```python
from build123d import *

# Parameters (mm, degrees)
CROQUIS3_R              = 6.25
CROQUIS3_R_2            = 4.25
SALIENTE_EXTRUIR1_DEPTH = 12
CORTAR_EXTRUIR1_DEPTH   = 10


with BuildPart() as part:
    # Croquis2 → Revolución1 (revolve)
    with BuildSketch(Plane.XY):
        Polygon((-4.25, 0), (-8, 7.5), (-10, 7.5), (-6.25, 0), align=None)
    revolve(axis=Axis((0, 7.5, 0), (0, -1, 0)))

    # Croquis3 → Saliente-Extruir1 (add)
    with BuildSketch(Plane.XZ):
        Circle(CROQUIS3_R)
        Circle(CROQUIS3_R_2, mode=Mode.SUBTRACT)
    extrude(amount=SALIENTE_EXTRUIR1_DEPTH)

    # Croquis4 → Cortar-Extruir1 (cut)
    with BuildSketch(Plane(origin=(0, 7.5, 0), x_dir=(1, 0, 0), z_dir=(0, 1, 0))):
        Polygon((-10.977061444, 8), (10.977061444, 8), (0, 12.60914387), align=None)
    extrude(amount=-CORTAR_EXTRUIR1_DEPTH, mode=Mode.SUBTRACT)


solid = part.part
```
The model under review builds one solid part; all positions refer to its coordinate system, in mm. A direction names the side the tool comes from. Give positions to 0.01 mm unless a question says otherwise; leave off trailing zeros. Write each loop counter-clockwise with the first axis right and the second up, starting at its lowest first coordinate (ties: lowest second). Pieces come first, ordered by that corner, then holes. Notation, with made-up numbers: M -23.5,-25.75 L 19.5,-25.75 A20 cw 19.5,-20.75 Z; hole C -24,40 d7. An arc over 180 degrees is marked long. Write each question's results on one line, items separated by ' | '. Start each with the question number.
1. For probe 1 along X at (y, z) = (-9.25, 0); probe 2 along X at (y, z) = (6.25, -1.25), list the stretches that pass through material, from the lowest coordinate up. Write a range as [from, to].
2. We need section A-A (z = 0). Write out the cut boundary in (x, y).
3. We need section B-B (y = -10.25). Write out the cut boundary in (x, z).
4. For faces 4 (the cylindrical face through (2.285, -5.916, 3.584)), 5 (the cylindrical face through (5.96, -5.92, 1.88)), list the 3-axis set-ups (+Z, -Z, +X, -X, +Y, -Y) from which the entire face can be reached by the end or side of a thin tool; tool diameter is ignored.
5. We need section C-C (y = 2.75). Write out the cut boundary in (x, z) (3 decimals), and give its area (3 significant figures).
6. Mouldability with a two-part tool opening along Z and no side actions: class faces 1 (the flat face through (0.7, 7.5, 8.3)), 2 (the conical face through (1.39, 0.36, 6.28)), 3 (the conical face through (-4.675, 1.302, -1.472)) as released by +Z, released by -Z, zero draft, split by the parting line, or undercut.
7. Insertion check: pin 1 Ø3 at (x, y) = (-6.5, 1) entering from +Z; pin 2 Ø3 at (x, z) = (2.5, 2) entering from +Y; pin 3 Ø7 at (x, z) = (0, 0) entering from -Y; pin 4 Ø1.5 at (x, y) = (7, 2.5) entering from -Z. Each pin has a flat end and moves straight along its axis. Give the tip position at first contact, or say it passes through.
Results found:
1) probe 1: x = [-6.25, -4.25], [4.25, 6.25] | probe 2: x = [-9.29, -7.27], [7.27, 9.29]
2) outline: M -10,7.5 L -6.25,0 L -6.25,-12 L -4.25,-12 L -4.25,0 L -8,7.5 Z; M 4.25,-12 L 6.25,-12 L 6.25,0 L 10,7.5 L 8,7.5 L 4.25,0 Z
3) outline: C 0,0 d12.5; hole C 0,0 d8.5
4) face 4: +Y, -Y | face 5: -Y
5) outline: C 0,0 d15.25; hole C 0,0 d11.25 | area: 83.3 mm^2
6) face 1: zero draft | face 2: split by the parting line | face 3: undercut
7) pin 1: stops at z = 4.88 | pin 2: stops at y = 0.9 | pin 3: passes through | pin 4: stops at z = -4.33
